Verification items for the finished model (mm, model axes). Face numbers are marked on the shaded views. Give positions to 0.01 mm unless a question says otherwise; leave off trailing zeros. Loops run counter-clockwise (first coordinate to the right, second up) from the corner with the lowest first, then second, coordinate; pieces in that order, holes last. Notation, with made-up numbers: (38, 8.25) - (90, 8.25) arc R31 ccw to (90, 38.25) - close; hole circle Ø3 at (81.5, -39.5). An arc over 180 degrees is marked (long way). Answer in a Markdown table with one row per item.
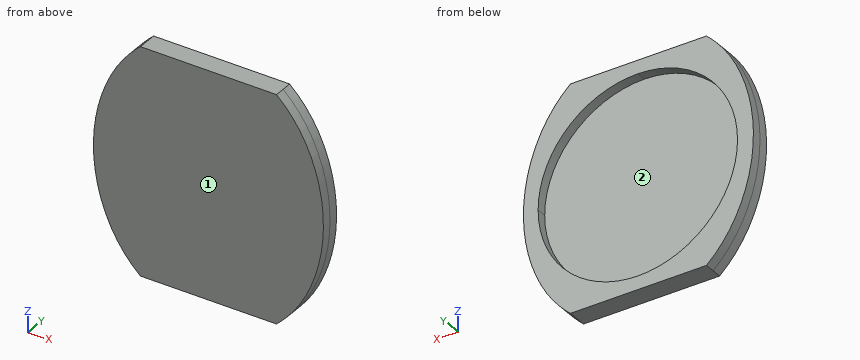
```python
from build123d import *

# Parameters (mm, degrees)
BOSS_EXTRUDE1_DEPTH     = 10
SKETCH1_3_R             = 100
BOSS_EXTRUDE2_DEPTH     = 10
SKETCH2_W               = 214.561996695
SKETCH2_H               = 67.979229187
CUT_EXTRUDE1_DEPTH      = 1.0000001
CUT_EXTRUDE1_DEPTH_BACK = 21.0000001


with BuildPart() as part:
    # Sketch1 → Boss-Extrude1 (new body, symmetric)
    with BuildSketch(Plane(origin=(0, 0, 0), x_dir=(1, 0, 0), z_dir=(0, 1, 0))):
        with BuildLine():
            add(Edge.make_bspline(
                [(0.976121303, -140.025549951), (2.374162629, -140.009491535), (3.771517421, -139.962591197), (7.291103261, -139.767278285), (9.398709168, -139.579437143), (15.675293836, -138.811953228), (19.799111475, -138.029795642), (27.929813311, -135.94328184), (31.936744561, -134.639135756), (37.859712235, -132.29247735), (39.804221595, -131.450894746), (43.623558737, -129.659192276), (45.500465995, -128.708195239), (51.0358335, -125.694698111), (54.599581786, -123.47277318), (59.764651016, -119.835967833), (61.45615035, -118.57288108), (63.948397978, -116.602501944), (64.77264308, -115.932207196), (66.398329816, -114.572915867), (67.200371286, -113.883479536), (71.15781434, -110.388473165), (74.15557851, -107.440023102), (79.839048175, -101.260277994), (82.526531921, -98.030594728), (86.325197715, -92.975281331), (87.552083684, -91.254523379), (89.92827313, -87.74268795), (91.071161278, -85.961213119), (93.264204581, -82.358005966), (94.315491716, -80.534886626), (96.329914932, -76.846718964), (97.291887312, -74.981117129), (100.057054093, -69.326876807), (101.744965365, -65.483403988), (104.050207299, -59.610400761), (104.780795243, -57.634741095), (106.166809965, -53.647671411), (106.823248507, -51.632689638), (108.669969422, -45.566700204), (109.738950442, -41.49400287), (111.566738836, -33.293705648), (112.32543315, -29.166085749), (113.538180225, -20.85692261), (113.992347502, -16.67539964), (114.36903765, -11.414684455), (114.434803631, -10.360847109), (114.547109075, -8.249769211), (114.593657534, -7.191844363), (114.703986475, -4.02388278), (114.738672, -1.916622031), (114.721208012, 8.596531177), (114.100106338, 16.933423498), (112.26337389, 29.32899767), (111.499343946, 33.442447781), (110.118494221, 39.584146802), (109.369324409, 42.647871971), (108.529677635, 45.700624473), (107.949499474, 47.733317125), (107.648881576, 48.749432437), (106.100547872, 53.802562864), (104.714467284, 57.768944772), (101.648347062, 65.549912048), (99.96820604, 69.364445062), (97.222621896, 74.969865164), (96.268251936, 76.818108957), (94.2727099, 80.469773084), (93.232568116, 82.273725448), (89.982350098, 87.618559335), (87.642859175, 91.092612835), (84.48192294, 95.313016777), (83.837654689, 96.150859096), (82.525451012, 97.814322319), (81.856640259, 98.64121338), (79.822125033, 101.093717437), (78.430527447, 102.688859664), (74.149311898, 107.353958125), (71.153616848, 110.303977016), (64.867354765, 115.870614214), (61.576656322, 118.487083942), (56.404777152, 122.145142784), (54.641398693, 123.31992646), (51.934089957, 125.011728379), (51.023681699, 125.562366877), (49.193658371, 126.632857883), (48.273010775, 127.153359084), (43.641538937, 129.682001779), (39.846190182, 131.469016566), (32.072993706, 134.565606006), (28.09510057, 135.875061848), (21.983291629, 137.459987939), (19.921721798, 137.924724312), (16.791518565, 138.522812496), (15.740120954, 138.705899718), (13.634978124, 139.036596855), (12.581020534, 139.184317529), (8.013946499, 139.747161721), (4.486924522, 139.985449555), (0.944318009, 140.025549951)],
                knots=[0.005345243, 0.005345243, 0.005345243, 0.005345243, 0.015625, 0.015625, 0.03125, 0.03125, 0.0625, 0.0625, 0.09375, 0.09375, 0.109375, 0.109375, 0.125, 0.125, 0.15625, 0.15625, 0.171875, 0.171875, 0.1796875, 0.1796875, 0.1875, 0.1875, 0.21875, 0.21875, 0.25, 0.25, 0.265625, 0.265625, 0.28125, 0.28125, 0.296875, 0.296875, 0.3125, 0.3125, 0.34375, 0.34375, 0.359375, 0.359375, 0.375, 0.375, 0.40625, 0.40625, 0.4375, 0.4375, 0.46875, 0.46875, 0.4765625, 0.4765625, 0.484375, 0.484375, 0.5, 0.5, 0.5625, 0.5625, 0.59375, 0.59375, 0.609375, 0.6171875, 0.6171875, 0.625, 0.625, 0.65625, 0.65625, 0.6875, 0.6875, 0.703125, 0.703125, 0.71875, 0.71875, 0.75, 0.75, 0.7578125, 0.7578125, 0.765625, 0.765625, 0.78125, 0.78125, 0.8125, 0.8125, 0.84375, 0.84375, 0.859375, 0.859375, 0.8671875, 0.8671875, 0.875, 0.875, 0.90625, 0.90625, 0.9375, 0.9375, 0.953125, 0.953125, 0.9609375, 0.9609375, 0.96875, 0.96875, 0.994746559, 0.994746559, 0.994746559, 0.994746559], degree=3))
            Line((0.944318009, 140.025549951), (0, 140.025549951))
            Line((0, 140.025549951), (0, 100))
            ThreePointArc((0, 100), (70.710678119, 70.710678119), (100, 0))
            ThreePointArc((100, 0), (70.710678119, -70.710678119), (0, -100))
            Line((0, -100), (0, -140.025549951))
            Line((0, -140.025549951), (0.976121303, -140.025549951))
        make_face()
        with BuildLine():
            Line((0, 100), (0, 140.025549951))
            add(Edge.make_bspline(
                [(0, 140.025549951), (-0.197417557, 140.027819409), (-0.394821383, 140.02947205), (-0.592211495, 140.030508539)],
                knots=[0, 0, 0, 0, 0.001450863, 0.001450863, 0.001450863, 0.001450863], degree=3))
            add(Edge.make_bspline(
                [(-0.592211495, 140.030508539), (-2.520604536, 140.040634466), (-4.447688548, 139.99195347), (-8.496389648, 139.767278285), (-10.603995555, 139.579437143), (-16.880580223, 138.811953228), (-21.004397862, 138.029795642), (-29.135099698, 135.94328184), (-33.142030948, 134.639135756), (-39.064998622, 132.29247735), (-41.009507982, 131.450894746), (-44.828845124, 129.659192276), (-46.705752383, 128.708195239), (-52.241119887, 125.694698111), (-55.804868173, 123.47277318), (-60.969937403, 119.835967833), (-62.661436737, 118.57288108), (-65.153684365, 116.602501944), (-65.977929468, 115.932207196), (-67.603616203, 114.572915867), (-68.405657673, 113.883479536), (-72.363100727, 110.388473165), (-75.360864897, 107.440023102), (-81.044334562, 101.260277994), (-83.731818308, 98.030594728), (-87.530484102, 92.975281331), (-88.757370071, 91.254523379), (-91.133559517, 87.74268795), (-92.276447665, 85.961213119), (-94.469490968, 82.358005966), (-95.520778103, 80.534886626), (-97.535201319, 76.846718964), (-98.497173699, 74.981117129), (-101.26234048, 69.326876807), (-102.950251753, 65.483403988), (-105.255493686, 59.610400761), (-105.98608163, 57.634741095), (-107.372096352, 53.647671411), (-108.028534894, 51.632689638), (-109.875255809, 45.566700204), (-110.944236829, 41.49400287), (-112.772025223, 33.293705648), (-113.530719537, 29.166085749), (-114.743466612, 20.85692261), (-115.197633889, 16.67539964), (-115.574324037, 11.414684455), (-115.640090018, 10.360847109), (-115.752395462, 8.249769211), (-115.798943921, 7.191844363), (-115.909272862, 4.02388278), (-115.943958388, 1.916622031), (-115.926494399, -8.596531177), (-115.305392725, -16.933423498), (-113.468660278, -29.32899767), (-112.704630333, -33.442447781), (-111.323780608, -39.584146802), (-110.574610796, -42.647871971), (-109.734964023, -45.700624473), (-109.154785861, -47.733317125), (-108.854167963, -48.749432437), (-107.305834259, -53.802562864), (-105.919753671, -57.768944772), (-102.85363345, -65.549912048), (-101.173492427, -69.364445062), (-98.427908283, -74.969865164), (-97.473538324, -76.818108957), (-95.477996287, -80.469773084), (-94.437854503, -82.273725448), (-91.187636485, -87.618559335), (-88.848145562, -91.092612835), (-85.687209327, -95.313016777), (-85.042941076, -96.150859096), (-83.730737399, -97.814322319), (-83.061926646, -98.64121338), (-81.02741142, -101.093717437), (-79.635813834, -102.688859664), (-75.354598285, -107.353958125), (-72.358903236, -110.303977016), (-66.072641152, -115.870614214), (-62.781942709, -118.487083942), (-57.610063539, -122.145142784), (-55.84668508, -123.31992646), (-53.139376344, -125.011728379), (-52.228968086, -125.562366877), (-50.398944758, -126.632857883), (-49.478297162, -127.153359084), (-44.846825324, -129.682001779), (-41.051476569, -131.469016566), (-33.278280093, -134.565606006), (-29.300386957, -135.875061848), (-23.188578016, -137.459987939), (-21.127008185, -137.924724312), (-17.996804952, -138.522812496), (-16.945407341, -138.705899718), (-14.840264511, -139.036596855), (-13.786306921, -139.184317529), (-8.711843514, -139.809692163), (-4.672693328, -140.050246998), (-0.613074893, -140.030508539)],
                knots=[0.001450863, 0.001450863, 0.001450863, 0.001450863, 0.015625, 0.015625, 0.03125, 0.03125, 0.0625, 0.0625, 0.09375, 0.09375, 0.109375, 0.109375, 0.125, 0.125, 0.15625, 0.15625, 0.171875, 0.171875, 0.1796875, 0.1796875, 0.1875, 0.1875, 0.21875, 0.21875, 0.25, 0.25, 0.265625, 0.265625, 0.28125, 0.28125, 0.296875, 0.296875, 0.3125, 0.3125, 0.34375, 0.34375, 0.359375, 0.359375, 0.375, 0.375, 0.40625, 0.40625, 0.4375, 0.4375, 0.46875, 0.46875, 0.4765625, 0.4765625, 0.484375, 0.484375, 0.5, 0.5, 0.5625, 0.5625, 0.59375, 0.59375, 0.609375, 0.6171875, 0.6171875, 0.625, 0.625, 0.65625, 0.65625, 0.6875, 0.6875, 0.703125, 0.703125, 0.71875, 0.71875, 0.75, 0.75, 0.7578125, 0.7578125, 0.765625, 0.765625, 0.78125, 0.78125, 0.8125, 0.8125, 0.84375, 0.84375, 0.859375, 0.859375, 0.8671875, 0.8671875, 0.875, 0.875, 0.90625, 0.90625, 0.9375, 0.9375, 0.953125, 0.953125, 0.9609375, 0.9609375, 0.96875, 0.96875, 0.998502653, 0.998502653, 0.998502653, 0.998502653], degree=3))
            add(Edge.make_bspline(
                [(-0.613074893, -140.030508539), (-0.408768455, -140.029515171), (-0.204410176, -140.027862544), (0, -140.025549951)],
                knots=[0.998502653, 0.998502653, 0.998502653, 0.998502653, 1, 1, 1, 1], degree=3))
            Line((0, -140.025549951), (0, -100))
            ThreePointArc((0, -100), (-100, 0), (0, 100))
        make_face()
    extrude(amount=BOSS_EXTRUDE1_DEPTH, both=True)

    # Sketch1<3> → Boss-Extrude2 (add)
    with BuildSketch(Plane(origin=(0, 0, 0), x_dir=(1, 0, 0), z_dir=(0, 1, 0))):
        Circle(SKETCH1_3_R)
        with BuildLine():
            ThreePointArc((100, 0), (70.710678119, 70.710678119), (0, 100))
            Line((0, 100), (0, -100))
            ThreePointArc((0, -100), (70.710678119, -70.710678119), (100, 0))
        make_face()
        with BuildLine():
            Line((0, -100), (0, 100))
            ThreePointArc((0, 100), (-100, 0), (0, -100))
        make_face()
    extrude(amount=-BOSS_EXTRUDE2_DEPTH)

    # Sketch2 → Cut-Extrude1 (cut, two sides)
    with BuildSketch(Plane(origin=(0, 10, 0), x_dir=(1, 0, 0), z_dir=(0, 1, 0))) as cut_extrude1_sk:
        with Locations((-8.659676613, -147.450639379)):
            Rectangle(SKETCH2_W, SKETCH2_H)
        with Locations((-8.659676613, 147.450639379)):
            Rectangle(SKETCH2_W, SKETCH2_H)
    extrude(amount=CUT_EXTRUDE1_DEPTH, mode=Mode.SUBTRACT)
    extrude(cut_extrude1_sk.sketch, amount=-CUT_EXTRUDE1_DEPTH_BACK, mode=Mode.SUBTRACT)


solid = part.part
```
Q1. Go/stop test with flat-tipped pins: P1, Ø1, axis at x = -76.5, y = -6, coming from the -Z side; P2, Ø6, axis at x = 40.5, z = -55.5, coming from the +Y side. Record where each tip stops, or that it passes through.
Completed:
| item | result |
|---|---|
| P1 | z = -106.68 |
| P2 | y = 0 |
Q2. Draft check along Z on the marked faces 1 and 2. Enter one of: +Z half, -Z half, draft (parallel to the pull), parting line (faces both ways), or undercut.
Completed:
| item | result |
|---|---|
| face 1 | draft |
| face 2 | undercut |
Q3. Sectioned sample at A-A (x = -62.5). Record the cut outline in (y, z), and give its area (3 significant figures).
Completed:
| item | result |
|---|---|
| outline | (-10, -113.46) - (10, -113.46) - (10, -78.06) - (0, -78.06) - (0, 78.06) - (10, 78.06) - (10, 113.46) - (-10, 113.46) - close |
| area | 2,980 mm^2 |
Q4. Sectioned sample at B-B (x = 21). Record the cut outline in (y, z).
Completed:
| item | result |
|---|---|
| outline | (-10, -113.46) - (10, -113.46) - (10, -97.77) - (0, -97.77) - (0, 97.77) - (10, 97.77) - (10, 113.46) - (-10, 113.46) - close |
Q5. Thickness scan on line 1 (Y direction, x = -14.5, z = 32); line 2 (X direction, y = 7.75, z = -6); line 3 (X direction, y = 4.5, z = 59). Record the ranges inside material, lowest first.
Completed:
| item | result |
|---|---|
| line 1 | -10 to 0 |
| line 2 | -115.84 to -99.82, 99.82 to 114.63 |
| line 3 | -105.41 to -80.74, 80.74 to 104.26 |
